from build123d import *

# Parameters (mm, degrees)
SKETCH1_R           = 2.4892
SKETCH1_R_2         = 10.16
BOSS_EXTRUDE1_DEPTH = 1.5875
FILLET1_R           = 3.175


with BuildPart() as part:
    # Sketch1 → Boss-Extrude1 (new, symmetric)
    with BuildSketch(Plane.XY):
        with BuildLine():
            Line((-25.4, 19.05), (0, 19.05))
            Line((0, 19.05), (25.4, 19.05))
            ThreePointArc((25.4, 19.05), (31.75, 0), (25.4, -19.05))
            Line((25.4, -19.05), (0, -19.05))
            Line((0, -19.05), (-25.4, -19.05))
            ThreePointArc((-25.4, -19.05), (-31.75, 0), (-25.4, 19.05))
        make_face()
        with Locations((21.997045256, 12.7)):
            Circle(SKETCH1_R, mode=Mode.SUBTRACT)
        with Locations((21.997045256, -12.7)):
            Circle(SKETCH1_R, mode=Mode.SUBTRACT)
        with Locations((-21.997045256, -12.7)):
            Circle(SKETCH1_R, mode=Mode.SUBTRACT)
        with Locations((-21.997045256, 12.7)):
            Circle(SKETCH1_R, mode=Mode.SUBTRACT)
        Circle(SKETCH1_R_2, mode=Mode.SUBTRACT)
    extrude(amount=BOSS_EXTRUDE1_DEPTH, both=True)

    # Fillet1
    fillet1_edges = [part.edges().sort_by_distance(p)[0] for p in [
        (-25.4, 19.05, 0),
        (25.4, 19.05, 0),
        (25.4, -19.05, 0),
        (-25.4, -19.05, 0),
    ]]
    fillet(fillet1_edges, radius=FILLET1_R)


solid = part.part
The listing builds one solid part. Answer for the finished solid, in the listing's coordinates (mm). Round coordinates to 2 decimals unless told otherwise and drop trailing zeros. Loops run counter-clockwise (first coordinate to the right, second up) from the corner with the lowest first, then second, coordinate; pieces in that order, holes last. Notation, with made-up numbers: M -21.75,27 L 19.25,27 A25 cw 19.25,41 Z; hole C 24.5,-38.75 d10. An arc over 180 degrees is marked long. Return JSON: item names as keys, results as strings.
Q1. This flat-tipped pin is pushed along its axis until it touches: pin 1 Ø1.5 at (y, z) = (-6, 0) entering from -X. Where does it stop, or does it pass through?
Results list:
{"pin 1": "stops at x = -31.31"}
Q2. Find section C-C, the plane z = -0.55. Determine the outline of the cut face in (x, y) (3 decimals), plus the area to 3 significant figures.
Results list:
{"outline": "M -26.399,-17.639 A3.175 ccw -23.76,-19.05 L 23.76,-19.05 A3.175 ccw 26.399,-17.639 A31.75 ccw 26.399,17.639 A3.175 ccw 23.76,19.05 L -23.76,19.05 A3.175 ccw -26.399,17.639 A31.75 ccw Z; hole C -21.997,-12.7 d4.978; hole C -21.997,12.7 d4.978; hole C 0,0 d20.32; hole C 21.997,-12.7 d4.978; hole C 21.997,12.7 d4.978", "area": "1,860 mm2"}
Q3. Find section D-D, the plane y = 12.7. Determine the outline of the cut face in (x, z).
Results list:
{"outline": "M -29.1,-1.59 L -24.49,-1.59 L -24.49,1.59 L -29.1,1.59 Z; M -19.51,-1.59 L 19.51,-1.59 L 19.51,1.59 L -19.51,1.59 Z; M 24.49,-1.59 L 29.1,-1.59 L 29.1,1.59 L 24.49,1.59 Z"}
Q4. The mould has two halves that part along Y. Classify faces 1 (the face through (-1.323, 10.074, -0.022)), 2 (the face through (31.75, 0.26, 0.02)), 3 (the face through (24.37, -11.95, -0.02)), 4 (the face through (-7, 9, -1.588)): released by +Y, released by -Y, zero draft, split by the parting line, or undercut.
Results list:
{"face 1": "undercut", "face 2": "split by the parting line", "face 3": "undercut", "face 4": "zero draft"}
Q5. Find the intervals of material crossed by line 1 along Y through (x, z) = (-20.5, -1); line 2 along X through (y, z) = (-10.5, -0.55); line 3 along Y through (x, z) = (20, 0.1), in increasing order. Write a range as from..to.
Results list:
{"line 1": "y = -19.05..-14.69, -10.71..10.71, 14.69..19.05", "line 2": "x = -29.96..-23.16, -20.83..20.83, 23.16..29.96", "line 3": "y = -19.05..-14.19, -11.21..11.21, 14.19..19.05"}
Q6. Find section A-A, the plane x = 0. Determine the outline of the cut face in (y, z), plus the area to 3 significant figures.
Results list:
{"outline": "M -19.05,-1.59 L -10.16,-1.59 L -10.16,1.59 L -19.05,1.59 Z; M 10.16,-1.59 L 19.05,-1.59 L 19.05,1.59 L 10.16,1.59 Z", "area": "56.5 mm2"}
Q7. Find section B-B, the plane y = 0. Determine the outline of the cut face in (x, z), plus the area to 3 significant figures.
Results list:
{"outline": "M -31.75,-1.59 L -10.16,-1.59 L -10.16,1.59 L -31.75,1.59 Z; M 10.16,-1.59 L 31.75,-1.59 L 31.75,1.59 L 10.16,1.59 Z", "area": "137 mm2"}
